Geometry check sheet. Reference: drawing and pictorial views, mm from the part's lowest x, y, z. Round coordinates to 2 decimals unless told otherwise and drop trailing zeros. Order: outer loops, then holes, each group sorted by start corner. A loop starts at its lowest first (then second) coordinate and runs counter-clockwise, first axis right, second up.
Q1. Depth check by flat-ended pin: P1, Ø2, axis at x = 97.5, z = 6, coming from the -Y side; P2, Ø2, axis at x = 36.5, z = 3, coming from the +Y side; P3, Ø5, axis at x = 94, z = 7, coming from the +Y side; P4, Ø3, axis at x = 103.75, y = 18.37, coming from the +Z side. Enter the tip coordinate at first touch or a pass-through.
Q2. Cross-section at A-A on y = 72.5. Record the cut outline in (x, z).
Q3. Cross-section at D-D on z = 3.5. Give the number of separate pieces and of enclosed holes in the cut face, then the cut area to 3 significant figures.
Q4. Scan lines: probe 1 along Y at (x, z) = (72.5, 8.75); probe 2 along Y at (x, z) = (43, 16) (1 decimal); probe 3 along X at (y, z) = (71.5, 19.25) (1 decimal). Record each from-to range of solid material in increasing order.
Q5. Mould release check, pull along X, two halves, no side actions. Record for the marked faces 1, 2 and 3: +X half, -X half, draft (parallel to the pull), parting line (faces both ways), or undercut.
Q6. Cross-section at C-C on x = 72.5. Record the cut outline in (y, z).
Q7. Cross-section at B-B on x = 103.75. Record the cut outline in (y, z).
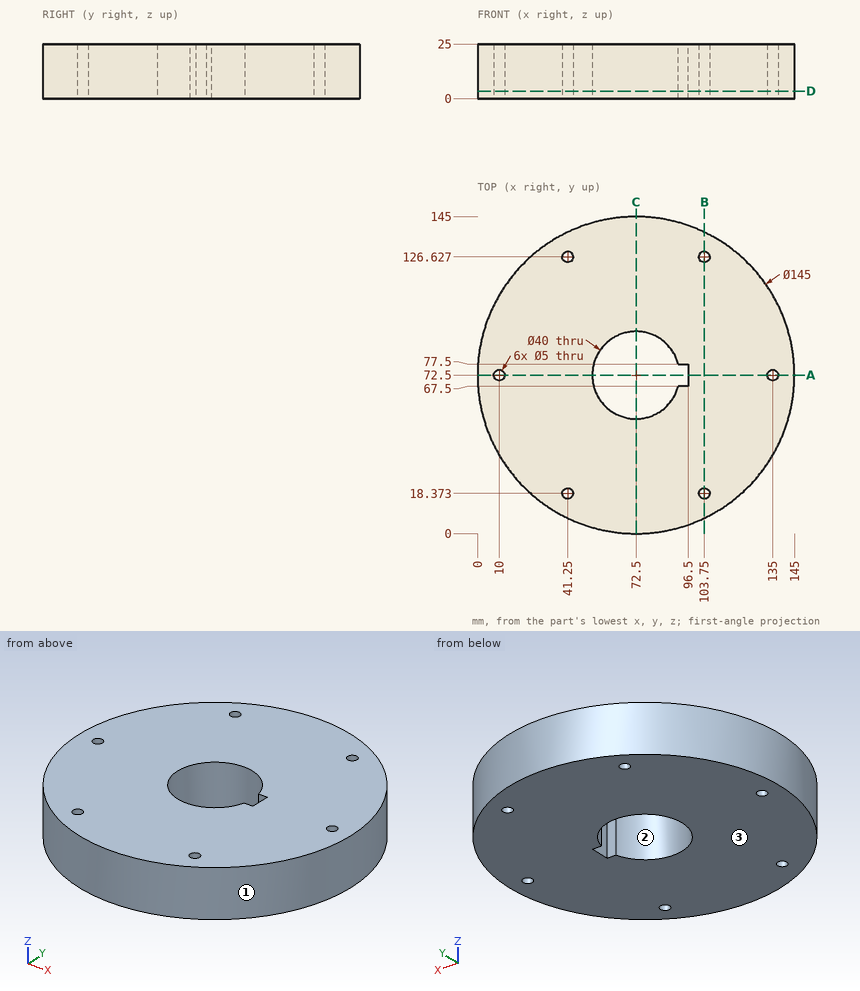
Results found:
1. P1: stops at y = 4.09
1. P2: stops at y = 135.99
1. P3: stops at y = 142.47
1. P4: passes through
2. outline: (0, 0) - (7.5, 0) - (7.5, 25) - (0, 25) - close; (12.5, 0) - (52.5, 0) - (52.5, 25) - (12.5, 25) - close; (96.5, 0) - (132.5, 0) - (132.5, 25) - (96.5, 25) - close; (137.5, 0) - (145, 0) - (145, 25) - (137.5, 25) - close
3. separate pieces: 1
3. enclosed holes: 7
3. area: 15,100 mm2
4. probe 1: y = 0 to 52.5, 92.5 to 145
4. probe 2: y = 6.3 to 16.6, 20.2 to 124.8, 128.4 to 138.7
4. probe 3: x = 0 to 7.7, 12.3 to 52.5, 96.5 to 132.7, 137.3 to 145
5. face 1: parting line
5. face 2: undercut
5. face 3: draft
6. outline: (0, 0) - (52.5, 0) - (52.5, 25) - (0, 25) - close; (92.5, 0) - (145, 0) - (145, 25) - (92.5, 25) - close
7. outline: (7.08, 0) - (15.87, 0) - (15.87, 25) - (7.08, 25) - close; (20.87, 0) - (124.13, 0) - (124.13, 25) - (20.87, 25) - close; (129.13, 0) - (137.92, 0) - (137.92, 25) - (129.13, 25) - close
